Autodesk Inventor part; units mm, degrees
ref_plane "Work Plane1" through (27.9676, -72.374, -408.43) normal (-1, 0, 0) x (0, 0, 1)
ref_plane "YZ Plane" through (0, 0, 0) normal (1, 0, 0) x (0, 1, 0)
ref_plane "XZ Plane" through (0, 0, 0) normal (0, 1, 0) x (-1, 0, 0)
sketch "Sketch1" plane through (0, 0, 0) normal (0, 0, 1) x (1, 0, 0)
  line L0 (-4.826, 0.413) -> (-4.826, -0.413)
  line L1 (-2.826, -2.413) -> (4.826, -2.413)
  line L2 (4.826, -2.413) -> (4.826, 2.413)
  line L3 (4.826, 2.413) -> (-2.826, 2.413)
  arc A0 (-4.826, -0.413) -> (-2.826, -2.413) centre (-2.826, -0.413) ccw
  arc A1 (-2.826, 2.413) -> (-4.826, 0.413) centre (-2.826, 0.413) ccw
  point P0 (0, 0)
extrude "Extrusion1" add sketch "Sketch1" along normal blind 10
sketch "Sketch2" plane through (4.826, -2.413, 0) normal (1, 0, 0) x (0, 0, -1)
  line L0 (0, 0) -> (-10, 0)
  line L1 (-10, 0) -> (-10, 4.826)
  circle A0 centre (3.175, 150.3292) radius 1.5
  circle A1 centre (3.175, 23.749) radius 1.5
  circle A2 centre (73.025, 23.749) radius 1.5
  circle A3 centre (73.025, 150.3292) radius 1.5
  arc A4 (60.2046, 236.2874) -> (0.9041, 211.5001) centre (77.9391, 110.5317) ccw
  ellipse E0 centre (170.686, 87.0391) end of major axis (408.43, 87.0391) minor radius 177.8 (0.9041, 211.5001) -> (0.9041, -37.4219) ccw
  arc A5 (0.9041, -37.4219) -> (60.2046, -62.2092) centre (77.9391, 63.5465) ccw
  arc A6 (60.2046, -62.2092) -> (281.1673, -62.2092) centre (170.686, 721.2179) ccw
  arc A7 (281.1673, -62.2092) -> (340.4678, -37.4219) centre (263.4329, 63.5465) ccw
  ellipse E1 centre (170.686, 87.0391) end of major axis (408.43, 87.0391) minor radius 177.8 (340.4678, -37.4219) -> (340.4678, 211.5001) ccw
  arc A8 (340.4678, 211.5001) -> (281.1673, 236.2874) centre (263.4329, 110.5317) ccw
  arc A9 (281.1673, 236.2874) -> (60.2046, 236.2874) centre (170.686, -547.1397) ccw
  circle A10 centre (18.1159, 118.5546) radius 1.25
  circle A11 centre (-51.7341, 53.7756) radius 1.25
  circle A12 centre (18.1159, 53.7756) radius 1.25
  circle A13 centre (-51.7341, 118.5546) radius 1.25
  circle A14 centre (395.605, 77.7641) radius 1.25
  circle A15 centre (321.1037, 62.7821) radius 1.25
  circle A16 centre (321.1037, 101.1361) radius 1.25
  circle A17 centre (395.605, 96.3141) radius 1.25
  line L2 (284.5488, 72.0792) -> (223.628, 72.0792)
  line L3 (223.628, 72.0792) -> (223.628, 102.5592)
  line L4 (223.628, 102.5592) -> (284.5488, 102.5592)
  line L5 (284.5488, 102.5592) -> (284.5488, 72.0792)
  circle A18 centre (129.4087, 87.0391) radius 30.4
  line L6 (95.6616, 45.3432) -> (95.6616, 49.3432)
  arc A19 (98.6614, 49.3432) -> (95.6616, 49.3432) centre (97.1615, 49.3432) ccw
  line L7 (98.6614, 49.3432) -> (98.6614, 45.3432)
  arc A20 (95.6616, 45.3432) -> (98.6614, 45.3432) centre (97.1615, 45.3432) ccw
  line L8 (160.3503, 45.3892) -> (160.3503, 49.3892)
  arc A21 (163.3501, 49.3892) -> (160.3503, 49.3892) centre (161.8502, 49.3892) ccw
  line L9 (163.3501, 49.3892) -> (163.3501, 45.3892)
  arc A22 (160.3503, 45.3892) -> (163.3501, 45.3892) centre (161.8502, 45.3892) ccw
  line L10 (95.5803, 159.8921) -> (95.5803, 163.8921)
  arc A23 (98.5801, 163.8921) -> (95.5803, 163.8921) centre (97.0802, 163.8921) ccw
  line L11 (98.5801, 163.8921) -> (98.5801, 159.8921)
  arc A24 (95.5803, 159.8921) -> (98.5801, 159.8921) centre (97.0802, 159.8921) ccw
  line L12 (163.3504, 163.8921) -> (163.3504, 159.8921)
  arc A25 (160.3506, 159.8921) -> (163.3504, 159.8921) centre (161.8505, 159.8921) ccw
  line L13 (160.3506, 159.8921) -> (160.3506, 163.8921)
  arc A26 (163.3504, 163.8921) -> (160.3506, 163.8921) centre (161.8505, 163.8921) ccw
  arc A27 (180.3755, 134.9774) -> (180.3753, 131.9798) centre (180.3755, 133.4786) ccw
  line L14 (180.3755, 134.9774) -> (184.3754, 134.9776)
  arc A28 (184.3754, 131.9796) -> (184.3754, 134.9776) centre (184.3755, 133.4786) ccw
  line L15 (184.3754, 131.9796) -> (180.3753, 131.9798)
  arc A29 (65.9852, 134.9725) -> (65.9851, 131.9749) centre (65.9852, 133.4737) ccw
  line L16 (65.9852, 134.9725) -> (69.9852, 134.9727)
  arc A30 (69.9852, 131.9747) -> (69.9852, 134.9727) centre (69.9852, 133.4737) ccw
  line L17 (69.9852, 131.9747) -> (65.9851, 131.9749)
  arc A31 (188.0254, 134.9778) -> (188.0255, 131.9802) centre (188.0255, 133.479) ccw
  line L18 (188.0254, 134.9778) -> (192.0254, 134.978)
  arc A32 (192.0254, 131.98) -> (192.0254, 134.978) centre (192.0255, 133.479) ccw
  line L19 (192.0254, 131.98) -> (188.0255, 131.9802)
  arc A33 (73.6382, 70.1265) -> (73.6381, 67.1289) centre (73.6382, 68.6277) ccw
  line L20 (73.6382, 70.1265) -> (77.6381, 70.1267)
  arc A34 (77.6381, 67.1287) -> (77.6381, 70.1267) centre (77.6382, 68.6277) ccw
  line L21 (77.6381, 67.1287) -> (73.6381, 67.1289)
  circle A35 centre (271.4412, 59.8872) radius 1.25
  circle A36 centre (229.978, 118.4342) radius 1.25
  circle A37 centre (281.3738, 108.9092) radius 1.25
  circle A38 centre (278.1988, 118.4342) radius 1.25
  circle A39 centre (254.0826, 118.4342) radius 1.25
  circle A40 centre (226.803, 108.9092) radius 1.25
  circle A41 centre (226.5872, 59.8872) radius 1.25
  arc A42 (188.0714, 70.2078) -> (188.0714, 67.2102) centre (188.0714, 68.709) ccw
  line L22 (188.0714, 70.2078) -> (192.0714, 70.208)
  arc A43 (192.0714, 67.21) -> (192.0714, 70.208) centre (192.0714, 68.709) ccw
  line L23 (192.0714, 67.21) -> (188.0714, 67.2102)
  line L24 (73.6352, 134.9725) -> (77.6351, 134.9727)
  arc A44 (77.6351, 131.9747) -> (77.6351, 134.9727) centre (77.6352, 133.4737) ccw
  line L25 (77.6351, 131.9747) -> (73.6351, 131.9749)
  arc A45 (73.6352, 134.9725) -> (73.6351, 131.9749) centre (73.6352, 133.4737) ccw
  arc A46 (66.0312, 70.1211) -> (66.0311, 67.1235) centre (66.0312, 68.6223) ccw
  line L26 (66.0312, 70.1211) -> (70.0312, 70.1213)
  arc A47 (70.0312, 67.1233) -> (70.0312, 70.1213) centre (70.0312, 68.6223) ccw
  line L27 (70.0312, 67.1233) -> (66.0311, 67.1235)
  arc A48 (180.4215, 70.2024) -> (180.4213, 67.2048) centre (180.4215, 68.7036) ccw
  line L28 (180.4215, 70.2024) -> (184.4214, 70.2025)
  arc A49 (184.4214, 67.2046) -> (184.4214, 70.2025) centre (184.4215, 68.7036) ccw
  line L29 (184.4214, 67.2046) -> (180.4213, 67.2048)
  line L30 (160.3503, 152.2421) -> (160.3503, 156.2421)
  arc A50 (163.3501, 156.2421) -> (160.3503, 156.2421) centre (161.8502, 156.2421) ccw
  line L31 (163.3501, 156.2421) -> (163.3501, 152.2421)
  arc A51 (160.3503, 152.2421) -> (163.3501, 152.2421) centre (161.8502, 152.2421) ccw
  line L32 (95.5857, 152.1961) -> (95.5857, 156.1961)
  arc A52 (98.5855, 156.1961) -> (95.5857, 156.1961) centre (97.0856, 156.1961) ccw
  line L33 (98.5855, 156.1961) -> (98.5855, 152.1961)
  arc A53 (95.5857, 152.1961) -> (98.5855, 152.1961) centre (97.0856, 152.1961) ccw
  line L34 (160.3503, 37.7392) -> (160.3503, 41.7392)
  arc A54 (163.3501, 41.7392) -> (160.3503, 41.7392) centre (161.8502, 41.7392) ccw
  line L35 (163.3501, 41.7392) -> (163.3501, 37.7392)
  arc A55 (160.3503, 37.7392) -> (163.3501, 37.7392) centre (161.8502, 37.7392) ccw
  line L36 (95.667, 37.6932) -> (95.667, 41.6932)
  arc A56 (98.6669, 41.6932) -> (95.667, 41.6932) centre (97.167, 41.6932) ccw
  line L37 (98.6669, 41.6932) -> (98.6669, 37.6932)
  arc A57 (95.667, 37.6932) -> (98.6669, 37.6932) centre (97.167, 37.6932) ccw
  line L38 (0, 4.826) -> (-10, 4.826)
  line L39 (0, -10.668) -> (0, 15.494)
  circle A58 centre (-5, -5.334) radius 1.5
  circle A59 centre (81.2, -5.334) radius 1.5
  circle A60 centre (81.2, 10.16) radius 1.5
  circle A61 centre (-5, 10.16) radius 1.5
  circle A62 centre (-5, 163.9182) radius 1.5
  circle A63 centre (81.2, 163.9182) radius 1.5
  circle A64 centre (81.2, 179.4122) radius 1.5
  circle A65 centre (-5, 179.4122) radius 1.5
  circle A66 centre (73.025, 187.9212) radius 1.5
  circle A67 centre (73.025, -13.843) radius 1.5
  circle A68 centre (3.175, -13.843) radius 1.5
  circle A69 centre (3.175, 187.9212) radius 1.5
  circle A70 centre (268.3469, 187.9212) radius 1.5
  circle A71 centre (260.1719, 179.4122) radius 1.5
  circle A72 centre (346.3719, 10.16) radius 1.5
  circle A73 centre (346.3719, -5.334) radius 1.5
  circle A74 centre (346.3719, 179.4122) radius 1.5
  circle A75 centre (338.1969, 150.3292) radius 1.5
  circle A76 centre (260.1719, -5.334) radius 1.5
  circle A77 centre (268.3469, 23.749) radius 1.5
  circle A78 centre (268.3469, -13.843) radius 1.5
  circle A79 centre (260.1719, 10.16) radius 1.5
  circle A80 centre (268.3469, 150.3292) radius 1.5
  circle A81 centre (338.1969, -13.843) radius 1.5
  circle A82 centre (338.1969, 23.749) radius 1.5
  circle A83 centre (260.1719, 163.9182) radius 1.5
  circle A84 centre (338.1969, 187.9212) radius 1.5
  circle A85 centre (346.3719, 163.9182) radius 1.25
  point P0 (0, 2.413)
ref_plane "Work Plane1" through (27.9676, -72.374, -408.43) normal (-1, 0, 0) x (0, 0, 1)
extrude "Extrusion2" add sketch "Sketch2" along normal up to surface (23.1416 mm away) contours L0 L1 L38 L39
sketch "Sketch3" plane through (27.9676, -2.413, 10) normal (1, 0, 0) x (0, 0, -1)
  line L0 (10, -10.668) -> (10, 15.494)
  line L1 (10, -10.668) -> (0, -10.668)
  line L2 (0, -10.668) -> (0, 15.494)
  line L3 (0, 15.494) -> (10, 15.494)
  line L4 (10, 15.494) -> (10, -10.668)
  line L5 (10, 2.826) -> (10, 2)
  line L6 (10, 0) -> (10, -10.668)
  line L7 (10, 4.826) -> (10, 15.494)
  circle A0 centre (5, -5.334) radius 1.25
  circle A1 centre (5, 10.16) radius 1.25
  point P0 (10, 2.413)
  point P1 (5, -10.668)
  point P2 (5, 15.494)
  point P3 (10, -5.334)
  point P4 (10, 10.16)
  dimension "d4" = 2.5
  dimension "d5" = 2.5
extrude "Extrusion3" add sketch "Sketch3" against normal blind 2
fillet "Fillet1" radius 1 6 edges at (25.9676, -2.413, 5) (25.9676, 2.413, 5) (26.9676, 13.081, 0) (26.9676, 13.081, 10) (26.9676, -13.081, 10) (26.9676, -13.081, 0)
sketch "Sketch4" plane through (0, 0, 10) normal (0, 0, 1) x (1, 0, 0)
  point P0 (0, 0)
sketch "Sketch5" plane through (0, 0, 10) normal (0, 0, 1) x (1, 0, 0)
  line L0 (27.9676, -12.081) -> (25.9676, -12.081)
  line L1 (27.9676, 12.081) -> (27.9676, -12.081)
  line L2 (25.9676, 12.081) -> (27.9676, 12.081)
  line L3 (25.9676, 3.413) -> (25.9676, 12.081)
  arc A0 (24.9676, 2.413) -> (25.9676, 3.413) centre (24.9676, 3.413) ccw
  line L4 (-2.826, 2.413) -> (24.9676, 2.413)
  arc A1 (-2.826, 2.413) -> (-4.826, 0.413) centre (-2.826, 0.413) ccw
  line L5 (-4.826, 0.413) -> (-4.826, -0.413)
  arc A2 (-4.826, -0.413) -> (-2.826, -2.413) centre (-2.826, -0.413) ccw
  line L6 (-2.826, -2.413) -> (24.9676, -2.413)
  arc A3 (25.9676, -3.413) -> (24.9676, -2.413) centre (24.9676, -3.413) ccw
  line L7 (25.9676, -12.081) -> (25.9676, -3.413)
  line L8 (-2.826, 2.413) -> (24.9676, 2.413)
  line L9 (-2.826, 2.413) -> (27.9676, 2.413)
  line L10 (27.9676, 2.413) -> (27.9676, -2.413)
  line L11 (27.9676, -2.413) -> (-2.826, -2.413)
  line L12 (-2.826, -2.413) -> (-2.826, 2.413)
  circle A4 centre (-2.826, 0.413) radius 2
  circle A5 centre (-2.826, -0.413) radius 2
  line L13 (-4.826, 0.413) -> (-4.826, -0.413)
  line L14 (-4.826, -0.413) -> (-4.826, 0.413)
  arc A6 (-2.826, 2.413) -> (-4.826, 0.413) centre (-2.826, 0.413) ccw
  point P0 (0, 0)
extrude "Extrusion4" add sketch "Sketch5" along normal blind 3 contours L11 L6 A5 A4 L4 L9 L1 | A2 A5 A4 L12 | L12 A4 A5 | L12 A5 A4 A1 | A4 A5 L12 | A4 A5 L12 | L12 A5 A4
sketch "Sketch6" plane through (-2.826, -2.413, 0) normal (0, -1, 0) x (1, 0, 0)
  line L0 (30.7936, 13) -> (0, 13)
  line L1 (30.7936, 10) -> (30.7936, 13)
  line L2 (30.7936, 13) -> (30.7936, 10)
  line L3 (30.7936, 10) -> (20.7936, 10)
  circle A0 centre (20.7936, 10) radius 1.5
  line L4 (20.7936, 10) -> (11.2936, 10)
  circle A1 centre (11.2936, 10) radius 1.5
  point P0 (2.826, 0)
  dimension "d11" = 10
  dimension "d12" = 3
  dimension "d13" = 9.5
  dimension "d14" = 3
extrude "Extrusion5" cut sketch "Sketch6" against normal blind 100
fillet "Fillet2" radius 1 4 edges at (12.5708, -2.413, 13) (-4.3794, -1.6728, 13) (12.5708, 2.413, 13) (-4.3794, 1.6728, 13)
properties part number "GuideArmConnector"
CAD build for the part. Positions are in the model's coordinates, mm. A direction names the side the tool comes from. Round coordinates to 2 decimals unless told otherwise and drop trailing zeros. Order: outer loops, then holes, each group sorted by start corner. A loop starts at its lowest first (then second) coordinate and runs counter-clockwise, first axis right, second up. Notation, with made-up numbers: (15, 62.25) - (33, 62.25) arc R20 ccw to (33, 77.25) - close; hole circle Ø2 at (12.5, -0.75). An arc over 180 degrees is marked (long way). Answer as CSV lines item,"result". Start each with the question number.
1. Pin check, flat tips, straight feed: pin 1 (3.5 mm diameter, centred on x = 27, y = -8, fed in from +Z); pin 2 (6 mm diameter, centred on x = 12, z = 7.5, fed in from +Y); pin 3 (3 mm diameter, centred on x = 14, y = -3.5, fed in from +Z); pin 4 (2 mm diameter, centred on y = 7.747, z = 5, fed in from -X). Stop position of each tip, or through.
2. Drill centre lines: L1, parallel to Y at x = 26.6, z = 5; L2, parallel to X at y = 1, z = 10.5; L3, parallel to Y at x = 10, z = 3.75. Where is each one in solid material? Low to high. Write a range as [from, to].
3. Saw through at A-A, the plane z = 5. Write the cut outline in (x, y), and give its area (3 significant figures).
4. Saw through at C-C, the plane x = 18. Write the cut outline in (y, z), and give its area (3 significant figures).
5. Saw through at B-B, the plane z = 3.25. Write the cut outline in (x, y).
6. Tool access for faces 5 (the face through (19.353, -0.034, 9.425)), 6 (the face through (27, 7, 10)), 7 (the face through (25.968, 9.4, 5.1)): list every direction of +Z, -Z, +X, -X, +Y, -Y with a clear straight run to the whole face (end or side of a thin tool).
7. Saw through at D-D, the plane y = -5.75. Write the cut outline in (x, z).
8. Pull direction Z, two halves, no side cores. Call faces 1 (the face through (27, -7, 10)), 2 (the face through (7.277, -0.034, 9.087)), 3 (the face through (26.954, 12.796, 0.301)), 4 (the face through (-4.826, 0, 5)): +Z half, -Z half, draft (parallel to the pull), parting line (faces both ways), or undercut.
Model answer:
1,pin 1,"stops at z = 10"
1,pin 2,"stops at y = 2.41"
1,pin 3,"stops at z = 12.81"
1,pin 4,"passes through"
2,L1,"y = [-13.08, -9], [-6.5, 6.5], [9, 13.08]"
2,L2,"x = [-4.74, 7.05], [9.88, 16.55], [19.38, 27.97]"
2,L3,"y = [-2.41, 2.41]"
3,outline,"(-4.83, -0.41) arc R2 ccw to (-2.83, -2.41) - (24.97, -2.41) arc R1 cw to (25.97, -3.41) - (25.97, -6.5) - (27.97, -6.5) - (27.97, 6.5) - (25.97, 6.5) - (25.97, 3.41) arc R1 cw to (24.97, 2.41) - (-2.83, 2.41) arc R2 ccw to (-4.83, 0.41) - close; (25.97, -13.08) - (27.97, -13.08) - (27.97, -9) - (25.97, -9) - close; (25.97, 9) - (27.97, 9) - (27.97, 13.08) - (25.97, 13.08) - close"
3,area,"190 mm²"
4,outline,"(-2.41, 0) - (2.41, 0) - (2.41, 8.5) - (-2.41, 8.5) - close; (-2.41, 11.5) - (2.41, 11.5) - (2.41, 12) arc R1 ccw to (1.41, 13) - (-1.41, 13) arc R1 ccw to (-2.41, 12) - close"
4,area,"47.8 mm²"
5,outline,"(-4.83, -0.41) arc R2 ccw to (-2.83, -2.41) - (24.97, -2.41) arc R1 cw to (25.97, -3.41) - (25.97, -13.08) - (27.97, -13.08) - (27.97, 13.08) - (25.97, 13.08) - (25.97, 3.41) arc R1 cw to (24.97, 2.41) - (-2.83, 2.41) arc R2 ccw to (-4.83, 0.41) - close"
6,face 5,"+Y, -Y"
6,face 6,"+Z, +X, -X, +Y"
6,face 7,"+Z, -Z, -X, +Y"
7,outline,"(25.97, 0) - (27.97, 0) - (27.97, 10) - (25.97, 10) - close"
8,face 1,"+Z half"
8,face 2,"undercut"
8,face 3,"-Z half"
8,face 4,"draft"
